Verification items for this drawing (mm, ordinates from the low corner). Coordinates: 2 decimals unless noted, no trailing zeros. Order: outer loops, then holes, each group sorted by start corner. A loop starts at its lowest first (then second) coordinate and runs counter-clockwise, first axis right, second up. Notation, with made-up numbers: (17.5, -27) -> (35.5, -27) arc R21 ccw to (35.5, 1) -> close; hole circle Ø9 at (5.5, -39.75). An arc over 180 degrees is marked (long way). Write each question's results on one line, items separated by ' | '. Start each with the question number.
(1) Cross-section at D-D on y = 34.5. Enter the section's corners in (x, z), and give its area (3 significant figures).
(2) Thickness scan on probe 1 along Y at (x, z) = (65, 2.4); probe 2 along X at (y, z) = (35, 2.6); probe 3 along Y at (x, z) = (66.5, 1.7). Record the ranges inside material, lowest first. Write a range as [from, to].
(3) Cross-section at C-C on z = 2.05. Give the number of separate pieces and of enclosed holes in the cut face, and give its area (3 significant figures).
(4) Cross-section at B-B on x = 25. Enter the section's corners in (y, z).
(5) Cross-section at A-A on y = 3. Enter the section's corners in (x, z), and give its area (3 significant figures).
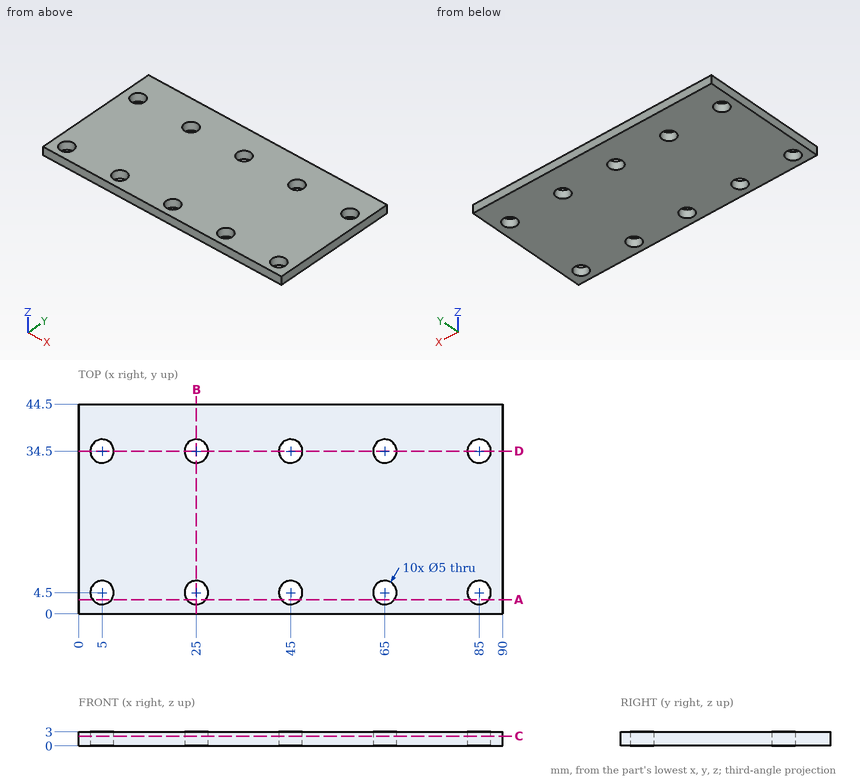
Results are:
1) outline: (0, 0) -> (2.5, 0) -> (2.5, 3) -> (0, 3) -> close; (7.5, 0) -> (22.5, 0) -> (22.5, 3) -> (7.5, 3) -> close; (27.5, 0) -> (42.5, 0) -> (42.5, 3) -> (27.5, 3) -> close; (47.5, 0) -> (62.5, 0) -> (62.5, 3) -> (47.5, 3) -> close; (67.5, 0) -> (82.5, 0) -> (82.5, 3) -> (67.5, 3) -> close; (87.5, 0) -> (90, 0) -> (90, 3) -> (87.5, 3) -> close | area: 195 mm2
2) probe 1: y = [0, 2], [7, 32], [37, 44.5] | probe 2: x = [0, 2.55], [7.45, 22.55], [27.45, 42.55], [47.45, 62.55], [67.45, 82.55], [87.45, 90] | probe 3: y = [0, 2.5], [6.5, 32.5], [36.5, 44.5]
3) separate pieces: 1 | enclosed holes: 10 | area: 3,810 mm2
4) outline: (0, 0) -> (2, 0) -> (2, 3) -> (0, 3) -> close; (7, 0) -> (32, 0) -> (32, 3) -> (7, 3) -> close; (37, 0) -> (44.5, 0) -> (44.5, 3) -> (37, 3) -> close
5) outline: (0, 0) -> (3, 0) -> (3, 3) -> (0, 3) -> close; (7, 0) -> (23, 0) -> (23, 3) -> (7, 3) -> close; (27, 0) -> (43, 0) -> (43, 3) -> (27, 3) -> close; (47, 0) -> (63, 0) -> (63, 3) -> (47, 3) -> close; (67, 0) -> (83, 0) -> (83, 3) -> (67, 3) -> close; (87, 0) -> (90, 0) -> (90, 3) -> (87, 3) -> close | area: 210 mm2
